The listing builds one solid part. Answer for the finished solid, in the listing's coordinates (mm). A direction names the side the tool comes from. Round coordinates to 2 decimals unless told otherwise and drop trailing zeros. Write each loop counter-clockwise with the first axis right and the second up, starting at its lowest first coordinate (ties: lowest second). Pieces come first, ordered by that corner, then holes.
Autodesk Inventor part; units mm, degrees
ref_plane "YZ Plane" through (0, 0, 0) normal (1, 0, 0) x (0, 1, 0)
ref_plane "XZ Plane" through (0, 0, 0) normal (0, 1, 0) x (-1, 0, 0)
ref_plane "XY Plane" through (0, 0, 0) normal (0, 0, 1) x (1, 0, 0)
sketch "Sketch1" plane through (0, 0, 0) normal (0, 0, 1) x (1, 0, 0)
  circle A0 centre (19.1135, 26.5479) radius 2.159
  circle A1 centre (6.4135, 13.8479) radius 2.159
  circle A2 centre (6.4135, 20.1979) radius 2.159
  circle A3 centre (19.1135, 13.8479) radius 2.159
  circle A4 centre (19.1135, 20.1979) radius 2.159
  circle A5 centre (-11.4935, -25.7761) radius 2.159
  circle A6 centre (-5.3048, -30.2218) radius 2.159
  circle A7 centre (-17.6822, -21.3304) radius 2.159
  arc A8 (2.921, 26.1944) -> (1.3335, 23.4448) centre (4.5085, 23.4448) ccw
  line L0 (1.3335, 23.4448) -> (1.3335, 14.8701)
  arc A9 (0.7371, 13.0177) -> (1.3335, 14.8701) centre (-1.8415, 14.8701) ccw
  line L1 (0.7371, 13.0177) -> (-21.808, -18.3666)
  arc A10 (-21.808, -18.3666) -> (-0.6209, -32.3394) centre (-11.4935, -25.7761) ccw
  line L2 (-0.6209, -32.3394) -> (23.7367, 8.0111)
  arc A11 (23.7367, 8.0111) -> (24.1935, 9.6519) centre (21.0185, 9.6519) ccw
  line L3 (24.1935, 9.6519) -> (24.1935, 32.9769)
  arc A12 (24.1935, 32.9769) -> (19.431, 35.7265) centre (21.0185, 32.9769) ccw
  line L4 (19.431, 35.7265) -> (2.921, 26.1944)
  circle A13 centre (21.0185, 9.6519) radius 3.175
  line L5 (1.3335, 14.8701) -> (1.3335, 13.8479)
  circle A14 centre (6.4135, 13.8479) radius 5.08
  line L6 (20.5313, 6.5145) -> (5.6339, 8.8281)
  circle A15 centre (-44.3865, 49.9375) radius 6.35
  circle A16 centre (-44.3865, 49.9375) radius 25.4 construction
  circle A17 centre (-11.4935, -25.7761) radius 82.55 construction
  circle A18 centre (-11.4935, -25.7761) radius 57.15 construction
  circle A19 centre (1.3335, 28.0719) radius 3.175
  line L7 (-1.8415, 28.0719) -> (-24.0665, 28.0719)
  circle A20 centre (-44.3865, 49.9375) radius 12.7
  line L8 (-24.0665, 28.0719) -> (-49.1272, 38.1555)
  line L9 (-39.4975, 61.6587) -> (22.2408, 35.9072)
  point P0 (0, 0)
  point P1 (1.6958, 24.9176)
  dimension "d10" = 6.35
  dimension "d3" = 12.7
  dimension "d4" = 50.8
  dimension "d5" = 114.3
  dimension "d6" = 45.72
  dimension "d8" = 25.4
  dimension "d12" = 1.524
  dimension "d13" = 25.4
extrude "Extrusion1" add sketch "Sketch1" along normal blind 3.175 contours A2 A14 L5 L0 A8 A19 L4 A12 L3 A13 A3 L6 | A2 A14 | A13 A3 A11 | L7 L8 A20 L9 A12 L4 A19 | A20 picked at (8.0498, 17.4208)
fillet "Fillet1" radius 3.175 3 edges at (1.6958, 24.9176, 1.5875) (-1.8415, 28.0719, 1.5875) (-24.0665, 28.0719, 1.5875)
properties part number "IntakePoly" material "Polycarbonate, Smoke"
1. Section B-B on y = 13 is taken. Determine the outline of the cut face in (x, z) (1 decimal), plus the area to 3 significant figures.
Geometry says:
outline: (1.4, 0) - (4.4, 0) - (4.4, 3.2) - (1.4, 3.2) - close; (8.4, 0) - (17.1, 0) - (17.1, 3.2) - (8.4, 3.2) - close; (21.1, 0) - (24.2, 0) - (24.2, 3.2) - (21.1, 3.2) - close
area: 47.1 mm2
2. Section A-A on x = 19 is taken. Determine the outline of the cut face in (y, z) (3 decimals), plus the area to 3 significant figures.
Geometry says:
outline: (6.752, 0) - (11.692, 0) - (11.692, 3.175) - (6.752, 3.175) - close; (16.004, 0) - (18.042, 0) - (18.042, 3.175) - (16.004, 3.175) - close; (22.354, 0) - (24.392, 0) - (24.392, 3.175) - (22.354, 3.175) - close; (28.704, 0) - (37.259, 0) - (37.259, 3.175) - (28.704, 3.175) - close
area: 55.8 mm2
3. Straight lines are drawn through the part: line 1 along X through (y, z) = (19.5, 2.45); line 2 along X through (y, z) = (12, 0.65); line 3 along Y through (x, z) = (8, 2.2). For each, find the intervals that lie inside material, in ascending order.
Geometry says:
line 1: x = 1.33 to 4.37, 8.46 to 17.07, 21.16 to 24.19
line 2: x = 1.68 to 5.3, 7.53 to 18, 20.23 to 24.19
line 3: y = 8.46 to 12.38, 15.31 to 18.73, 21.66 to 41.85
4. Section D-D on y = 41.5 is taken. Determine the outline of the cut face in (x, z) (3 decimals), plus the area to 3 significant figures.
Geometry says:
outline: (-53.879, 0) - (8.832, 0) - (8.832, 3.175) - (-53.879, 3.175) - close
area: 199 mm2
5. A tool of negligible diameter and unlimited length cuts with its end or side. For faces 1 (the face through (1.334, 18, 2)), 2 (the face through (-9.061, 48.963, 1.565)), from which of +Z, -Z, +X, -X, +Y, -Y can it reach the whole face along a straight path? Write none if from no direction.
Geometry says:
face 1: +Z, -Z, -X, -Y
face 2: +Z, -Z, +X, +Y
6. Given pin 1 (5 mm diameter, centred on x = 6.41, y = 13.85, fed in from -Z); pin 2 (1.5 mm diameter, centred on x = -35, z = 0.5, fed in from +Y); pin 3 (1 mm diameter, centred on x = -11, z = 1.5, fed in from -Y), each flat-ended and moving along its own axis, determine where each tip first touches the part or whether it passes through.
Geometry says:
pin 1: stops at z = 0
pin 2: stops at y = 60.1
pin 3: stops at y = 28.07
7. For a pull along Y with two mould halves and no side action, classify faces 3 (the face through (-50.73, 49.66, 1.57)), 4 (the face through (24.08, 8.81, 1.57)), 5 (the face through (-17, 35, 0)) as released by +Y, released by -Y, zero draft, split by the parting line, or undercut.
Geometry says:
face 3: undercut
face 4: released by -Y
face 5: zero draft
8. Section C-C on x = -43 is taken. Determine the outline of the cut face in (y, z) (3 decimals), plus the area to 3 significant figures.
Geometry says:
outline: (35.69, 0) - (43.741, 0) - (43.741, 3.175) - (35.69, 3.175) - close; (56.134, 0) - (62.562, 0) - (62.562, 3.175) - (56.134, 3.175) - close
area: 46.0 mm2
